```python
from build123d import *

# Parameters (mm, degrees)
F0_R     = 4.8745106906
F1_DEPTH = 25.4


with BuildPart() as f1:
    # F0 (on Front) → F1 (new body)
    with BuildSketch(Plane.XZ):
        with BuildLine():
            ThreePointArc((-9.4502929642, 115.490625), (-0.596483242, 104.7936951058), (9.525, 114.3))
            ThreePointArc((9.525, 114.3), (9.5063048942, 114.896483242), (9.4502929642, 115.490625))
            ThreePointArc((9.4502929642, 115.490625), (0, 123.825), (-9.4502929642, 115.490625))
        make_face()
        with Locations((0, 114.3)):
            Circle(F0_R, mode=Mode.SUBTRACT)
        with BuildLine():
            ThreePointArc((9.4502929642, 115.490625), (9.5063048942, 114.896483242), (9.525, 114.3))
            ThreePointArc((9.525, 114.3), (-0.596483242, 104.7936951058), (-9.4502929642, 115.490625))
            Line((-9.4502929642, 115.490625), (-15.7504882737, 65.484375))
            ThreePointArc((-15.7504882737, 65.484375), (0, 79.375), (15.7504882737, 65.484375))
            Line((15.7504882737, 65.484375), (9.4502929642, 115.490625))
        make_face()
        with Locations((-4.8745106906, 98.495259881)):
            Circle(F0_R, mode=Mode.SUBTRACT)
        with BuildLine():
            ThreePointArc((15.875, 63.5), (15.8438414904, 64.4941387366), (15.7504882737, 65.484375))
            ThreePointArc((15.7504882737, 65.484375), (0, 79.375), (-15.7504882737, 65.484375))
            ThreePointArc((-15.7504882737, 65.484375), (-15.8737438155, 63.6997054867), (-15.7954255641, 61.9125))
            ThreePointArc((-15.7954255641, 61.9125), (0, 47.625), (15.7954255641, 61.9125))
            ThreePointArc((15.7954255641, 61.9125), (15.8550939106, 62.7052534459), (15.875, 63.5))
        make_face()
        with Locations((0, 63.5)):
            Circle(F0_R, mode=Mode.SUBTRACT)
        with BuildLine():
            ThreePointArc((15.7954255641, 61.9125), (0, 47.625), (-15.7954255641, 61.9125))
            Line((-15.7954255641, 61.9125), (-9.4772553384, -0.9525))
            ThreePointArc((-9.4772553384, -0.9525), (-6.948684782, 6.5147068085), (0.3401785714, 9.5189234444))
            Line((0.3401785714, 9.5189234444), (10.4932062399, 9.1560838367))
            Line((10.4932062399, 9.1560838367), (15.7954255641, 61.9125))
        make_face()
        with BuildLine():
            ThreePointArc((0.3401785714, 9.5189234444), (-6.948684782, 6.5147068085), (-9.4772553384, -0.9525))
            ThreePointArc((-9.4772553384, -0.9525), (-6.2623833816, -7.1769199091), (0.3401785714, -9.5189234444))
            ThreePointArc((0.3401785714, -9.5189234444), (6.5147068085, -6.948684782), (9.4772553384, -0.9525))
            ThreePointArc((9.4772553384, -0.9525), (9.5130563464, -0.4768479324), (9.525, 0))
            ThreePointArc((9.525, 0), (6.8544082857, 6.6138273378), (0.3401785714, 9.5189234444))
        make_face()
        Circle(F0_R, mode=Mode.SUBTRACT)
        with BuildLine():
            Line((44.7334821429, 7.9324362036), (10.4932062399, 9.1560838367))
            Line((10.4932062399, 9.1560838367), (9.4772553384, -0.9525))
            ThreePointArc((9.4772553384, -0.9525), (6.5147068085, -6.948684782), (0.3401785714, -9.5189234444))
            Line((0.3401785714, -9.5189234444), (44.7334821429, -7.9324362036))
            ThreePointArc((44.7334821429, -7.9324362036), (36.5125, 0), (44.7334821429, 7.9324362036))
        make_face()
        with BuildLine():
            Line((9.4772553384, -0.9525), (10.4932062399, 9.1560838367))
            Line((10.4932062399, 9.1560838367), (0.3401785714, 9.5189234444))
            ThreePointArc((0.3401785714, 9.5189234444), (6.8544082857, 6.6138273378), (9.525, 0))
            ThreePointArc((9.525, 0), (9.5130563464, -0.4768479324), (9.4772553384, -0.9525))
        make_face()
        with BuildLine():
            ThreePointArc((52.3875, 0), (50.1620069047, 5.5115227815), (44.7334821429, 7.9324362036))
            ThreePointArc((44.7334821429, 7.9324362036), (36.5125, 0), (44.7334821429, -7.9324362036))
            ThreePointArc((44.7334821429, -7.9324362036), (50.1620069047, -5.5115227815), (52.3875, 0))
        make_face()
        with Locations((44.45, 0)):
            Circle(F0_R, mode=Mode.SUBTRACT)
    extrude(amount=F1_DEPTH)


solid = f1.part
```
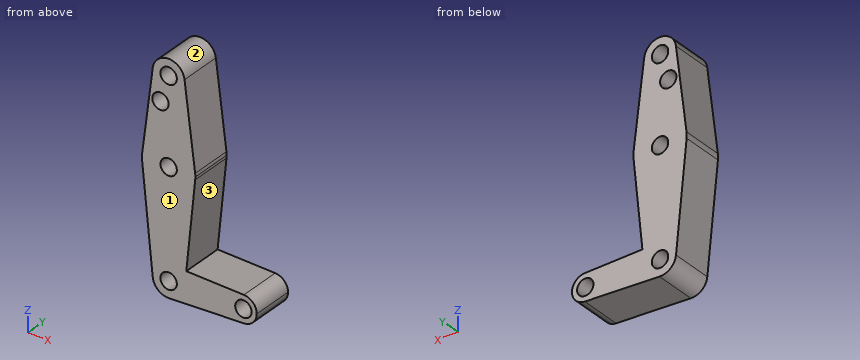
Read the model definition and answer for the solid it produces. Units are mm, in the model's axes. Face numbers are marked on the shaded views. Round coordinates to 2 decimals unless told otherwise and drop trailing zeros. Write each loop counter-clockwise with the first axis right and the second up, starting at its lowest first coordinate (ties: lowest second). Pieces come first, ordered by that corner, then holes. Notation, with made-up numbers: (-6, -37) - (-1, -37) arc R14 cw to (-1, -23) - close; hole circle Ø10 at (-11.75, -3). An arc over 180 degrees is marked (long way). Use CSV: the item, a comma, the result in double quotes.
Q1. Find section B-B, the plane y = -18.5. Count the separate pieces of the cut face and the enclosed holes in it, then the cut area to 3 significant figures.
Values:
separate pieces,"1"
enclosed holes,"5"
area,"3,540 mm²"
Q2. Find section A-A, the plane x = 12.5. Write down the section's boundary in (y, z), then the cut area to 3 significant figures.
Values:
outline,"(-25.4, -9.08) - (0, -9.08) - (0, 9.08) - (-25.4, 9.08) - close; (-25.4, 29.12) - (0, 29.12) - (0, 91.28) - (-25.4, 91.28) - close"
area,"2,040 mm²"
Q3. Each of these flat-tipped pins is pushed along its axis until it touches: pin 1 Ø2 at (x, y) = (22, -10.5) entering from -Z; pin 2 Ø5 at (x, y) = (9, -9) entering from +Z; pin 3 Ø8 at (y, z) = (-20.5, 81.5) entering from -X. Where does it stop, or does it pass through?
Values:
pin 1,"stops at z = -8.78"
pin 2,"stops at z = 121.26"
pin 3,"stops at x = -14.24"
Q4. Find section C-C, the plane z = 37. Write down the section's boundary in (x, y), then the cut area to 3 significant figures.
Values:
outline,"(-13.29, -25.4) - (13.29, -25.4) - (13.29, 0) - (-13.29, 0) - close"
area,"675 mm²"
Q5. Straight lines are drawn through the part: line 1 along Z through (x, y) = (46.5, -17.25); line 2 along Z through (x, y) = (44.45, -20); line 3 along X through (y, z) = (-19.5, 62). For each, find the intervals that lie inside material, in ascending order.
Values:
line 1,"z = -7.67 to -4.42, 4.42 to 7.67"
line 2,"z = -7.94 to -4.87, 4.87 to 7.94"
line 3,"x = -15.8 to -4.64, 4.64 to 15.8"
Q6. Determine the mould class of the marked faces 1, 2 and 3 for opening direction Z: +Z half, -Z half, draft (parallel to the pull), parting line (faces both ways), or undercut.
Values:
face 1,"draft"
face 2,"+Z half"
face 3,"undercut"
